```python
from build123d import *

# Parameters (mm, degrees)
CROQUIS1_W              = 50
CROQUIS1_H              = 50
SALIENTE_EXTRUIR1_DEPTH = 5
CROQUIS2_W              = 13
CROQUIS2_H              = 6
SALIENTE_EXTRUIR2_DEPTH = 9
CROQUIS3_R              = 2.5
CORTAR_EXTRUIR5_DEPTH   = 58.628118137
REDONDEO1_R             = 2
CORTAR_EXTRUIR6_DEPTH   = 4
CROQUIS5_R              = 1.5
CORTAR_EXTRUIR7_DEPTH   = 4


with BuildPart() as part:
    # Croquis1 → Saliente-Extruir1 (new body)
    with BuildSketch(Plane.XY):
        Rectangle(CROQUIS1_W, CROQUIS1_H)
        with BuildLine():
            Line((7, -16), (-7, -16))
            ThreePointArc((-7, -16), (-10.535533906, -14.535533906), (-12, -11))
            Line((-12, -11), (-12, 11))
            ThreePointArc((-12, 11), (-10.535533906, 14.535533906), (-7, 16))
            Line((-7, 16), (7, 16))
            ThreePointArc((7, 16), (10.535533906, 14.535533906), (12, 11))
            Line((12, 11), (12, -11))
            ThreePointArc((12, -11), (10.535533906, -14.535533906), (7, -16))
        make_face(mode=Mode.SUBTRACT)
    extrude(amount=SALIENTE_EXTRUIR1_DEPTH)

    # Croquis2 → Saliente-Extruir2 (add)
    with BuildSketch(Plane.XY.offset(5)):
        with Locations((18.5, 22)):
            Rectangle(CROQUIS2_W, CROQUIS2_H)
        with Locations((-18.5, 22)):
            Rectangle(CROQUIS2_W, CROQUIS2_H)
        with Locations((18.5, -22)):
            Rectangle(CROQUIS2_W, CROQUIS2_H)
        with Locations((-18.5, -22)):
            Rectangle(CROQUIS2_W, CROQUIS2_H)
    extrude(amount=SALIENTE_EXTRUIR2_DEPTH)

    # Croquis3 → Cortar-Extruir5 (cut, through all)
    with BuildSketch(Plane(origin=(0, 25, 0), x_dir=(1, 0, 0), z_dir=(0, 1, 0))):
        with Locations(Location((-18.5, -11.45, 0), (0, 0, 180))):
            Circle(CROQUIS3_R)
        with Locations(Location((18.5, -11.45, 0), (0, 0, 90))):
            Circle(CROQUIS3_R)
    extrude(amount=-CORTAR_EXTRUIR5_DEPTH, mode=Mode.SUBTRACT)

    # Redondeo1
    redondeo1_edges = [part.edges().sort_by_distance(p)[0] for p in [
        (-12, 22, 5),
        (12, 22, 5),
        (12, -22, 5),
        (-12, -22, 5),
    ]]
    fillet(redondeo1_edges, radius=REDONDEO1_R)

    # Croquis4 → Cortar-Extruir6 (cut)
    with BuildSketch(Plane.XY.offset(5)):
        Polygon((-1.010362971, 18.75), (1.010362971, 18.75), (2.020725942, 20.5), (1.010362971, 22.25), (-1.010362971, 22.25), (-2.020725942, 20.5), align=None)
        Polygon((-2.020725942, -20.5), (-1.010362971, -18.75), (1.010362971, -18.75), (2.020725942, -20.5), (1.010362971, -22.25), (-1.010362971, -22.25), align=None)
    extrude(amount=-CORTAR_EXTRUIR6_DEPTH, mode=Mode.SUBTRACT)

    # Croquis5 → Cortar-Extruir7 (cut)
    with BuildSketch(Plane.XY.offset(1)):
        with Locations((0, 20.5)):
            Circle(CROQUIS5_R)
        with Locations((0, -20.5)):
            Circle(CROQUIS5_R)
    extrude(amount=-CORTAR_EXTRUIR7_DEPTH, mode=Mode.SUBTRACT)


solid = part.part
```
The listing builds one solid part. Answer for the finished solid, in the listing's coordinates (mm). A direction names the side the tool comes from. Give positions to 0.01 mm unless a question says otherwise; leave off trailing zeros. Write each loop counter-clockwise with the first axis right and the second up, starting at its lowest first coordinate (ties: lowest second). Pieces come first, ordered by that corner, then holes. Notation, with made-up numbers: M 40.25,-2.5 L 52.25,-2.5 A9 cw 52.25,6.5 Z; hole C 13.5,27 d11. An arc over 180 degrees is marked long. Write each question's results on one line, items separated by ' | '.
Q1. Section C-C, the plane z = 11.45 is taken. Count the separate pieces of the cut face and the enclosed holes in it, then the cut area to 3 significant figures.
Output values:
separate pieces: 8 | enclosed holes: 0 | area: 192 mm2
Q2. For a pull along X with two mould halves and no side action, classify faces 5 (the flat face through (-18, 19, 8)), 6 (the flat face through (-1.5, -21.4, 3)) as released by +X, released by -X, zero draft, split by the parting line, or undercut.
Output values:
face 5: zero draft | face 6: undercut
Q3. Section D-D, the plane y = 15 is taken. Write down the section's boundary in (x, z), then the cut area to 3 significant figures.
Output values:
outline: M -25,0 L -10,0 L -10,5 L -25,5 Z; M 10,0 L 25,0 L 25,5 L 10,5 Z | area: 150 mm2
Q4. Section A-A, the plane x = 0 is taken. Write down the section's boundary in (y, z), then the cut area to 3 significant figures.
Output values:
outline: M -25,0 L -22,0 L -22,1 L -22.25,1 L -22.25,5 L -25,5 Z; M -19,0 L -16,0 L -16,5 L -18.75,5 L -18.75,1 L -19,1 Z; M 16,0 L 19,0 L 19,1 L 18.75,1 L 18.75,5 L 16,5 Z; M 22,0 L 25,0 L 25,5 L 22.25,5 L 22.25,1 L 22,1 Z | area: 56.0 mm2
Q5. Consider L1, parallel to Y at x = 0, z = 0.35; L2, parallel to X at y = -21, z = 8.5; L3, parallel to Y at x = 12.5, z = 13.25. Determine where each line is inside the solid, lowest interval first. Write a range as from..to.
Output values:
L1: -25..-22, -19..-16, 16..19, 22..25 | L2: -25..-12, 12..25 | L3: -25..-19, 19..25
Q6. A tool of negligible diameter and unlimited length cuts with its end or side. For faces 1 (the flat face through (0, -22.25, 3)), 2 (the cylindrical face through (-11.4, -21.96, 5.57)), 3 (the flat face through (0, -16, 2)), 4 (the flat face through (17, -19, 8)), from which of +Z, -Z, +X, -X, +Y, -Y can it reach the whole face along a straight path? Write none if from no direction.
Output values:
face 1: +Z | face 2: +Z, +Y, -Y | face 3: +Z, -Z | face 4: +Z, +X, -X
Q7. Section B-B, the plane z = 8 is taken. Write down the section's boundary in (x, y), then the cut area to 3 significant figures.
Output values:
outline: M -25,-25 L -12,-25 L -12,-19 L -25,-19 Z; M -25,19 L -12,19 L -12,25 L -25,25 Z; M 12,-25 L 25,-25 L 25,-19 L 12,-19 Z; M 12,19 L 25,19 L 25,25 L 12,25 Z | area: 312 mm2
Q8. Flat-ended cylindrical pins translate along their axes: P1, Ø2, axis at x = -17.5, y = -14.5, coming from the -Z side; P2, Ø10, axis at x = -6, y = -8.5, coming from the -Z side; P3, Ø3, axis at x = 12, y = -9.5, coming from the +Z side. Find the tip coordinate at first contact, or state that the pin passes through.
Output values:
P1: z = 0 | P2: through | P3: z = 5
